Model file for the job. Use its own axes, mm. Round coordinates to 2 decimals unless told otherwise and drop trailing zeros. Order: outer loops, then holes, each group sorted by start corner. A loop starts at its lowest first (then second) coordinate and runs counter-clockwise, first axis right, second up. Notation, with made-up numbers: (68.25, -15.75) -> (86.25, -15.75) arc R20 ccw to (86.25, -10.75) -> close; hole circle Ø9 at (68.25, 82). An arc over 180 degrees is marked (long way). Use CSV: the item, a comma, the result in double quotes.
```python
from build123d import *

# Parameters (mm, degrees)
SKETCH1_R               = 50.8
SKETCH1_R_2             = 48.7934
BOSS_EXTRUDE1_DEPTH     = 304.8
CUT_EXTRUDE1_REACH      = 327.279
CUT_EXTRUDE1_END_RADIUS = 48.7934
SKETCH2_R               = 1.651
CIRPATTERN1_COUNT       = 4


with BuildPart() as part:
    # Sketch1 → Boss-Extrude1 (new body)
    with BuildSketch(Plane.XY):
        with Locations(Location((0, 0, 0), (0, 0, 180))):
            Circle(SKETCH1_R)
        with Locations(Location((0, 0, 0), (0, 0, 180))):
            Circle(SKETCH1_R_2, mode=Mode.SUBTRACT)
    extrude(amount=BOSS_EXTRUDE1_DEPTH)

    # Cut-Extrude1: up to this cylinder (the profile starts outside it)
    cut_extrude1_end = Plane(origin=(0, 0, 196.85), z_dir=(0, 0, -1)) * Cylinder(CUT_EXTRUDE1_END_RADIUS, 753.1448, mode=Mode.PRIVATE)
    # Sketch2 → Cut-Extrude1 (cut, up to the surface)
    with BuildSketch(Plane.ZY.offset(50.8), mode=Mode.PRIVATE) as cut_extrude1_sk1:
        with Locations((196.85, 0)):
            Circle(SKETCH2_R)
    cut_extrude1_tool1 = extrude(cut_extrude1_sk1.sketch, amount=-CUT_EXTRUDE1_REACH, mode=Mode.PRIVATE) - cut_extrude1_end
    cut_extrude1 = cut_extrude1_tool1.solids().sort_by_distance((-50.8, 0, 196.85))[0]
    add(cut_extrude1, mode=Mode.SUBTRACT)

    # CirPattern1: Cut-Extrude1 ×4 about axis
    cirpattern1_axis = Axis((0, 0, 304.8), (0, 0, -1))
    for i in range(1, CIRPATTERN1_COUNT):
        add(cut_extrude1.rotate(cirpattern1_axis, i * 360 / CIRPATTERN1_COUNT), mode=Mode.SUBTRACT)


solid = part.part
```
Q1. Cut at C-C (z = 117). Give the cut face in (x, y).
From the geometry:
outline,"circle Ø101.6 at (0, 0); hole circle Ø97.59 at (0, 0)"
Q2. Cut at B-B (x = 30.5). Give the cut face in (y, z) (3 decimals).
From the geometry:
outline,"(-40.625, 0) -> (-38.086, 0) -> (-38.086, 304.8) -> (-40.625, 304.8) -> close; (38.086, 0) -> (40.625, 0) -> (40.625, 304.8) -> (38.086, 304.8) -> close"
Q3. Cut at A-A (y = -8). Give the cut face in (x, z).
From the geometry:
outline,"(-50.17, 0) -> (-48.13, 0) -> (-48.13, 304.8) -> (-50.17, 304.8) -> close; (48.13, 0) -> (50.17, 0) -> (50.17, 304.8) -> (48.13, 304.8) -> close"
Q4. Probe line 1 along Z through (x, y) = (0, 49); line 2 along Y through (x, z) = (-37, 248.5); line 3 along Y through (x, z) = (-27, 287.5). List the from-to ranges inside material, lowest first.
From the geometry:
line 1,"z = 0 to 195.2, 198.5 to 304.8"
line 2,"y = -34.81 to -31.81, 31.81 to 34.81"
line 3,"y = -43.03 to -40.64, 40.64 to 43.03"
Q5. Pin check, flat tips, straight feed: pin 1 (2 mm diameter, centred on y = 0, z = 196.85, fed in from -X); pin 2 (1 mm diameter, centred on x = -7, z = 58, fed in from -Y); pin 3 (1 mm diameter, centred on x = 23, z = 179.5, fed in from +Y); pin 4 (6 mm diameter, centred on y = -26, z = 153, fed in from -X). Stop position of each tip, or through.
From the geometry:
pin 1,"passes through"
pin 2,"stops at y = -50.38"
pin 3,"stops at y = 45.55"
pin 4,"stops at x = -45.3"
